```python
from build123d import *

# Parameters (mm, degrees)
SKETCH1_W              = 20
SKETCH1_H              = 50
BOSS_EXTRUDE1_DEPTH    = 15
SKETCH3_W              = 20
SKETCH3_H              = 50
BOSS_EXTRUDE2_DEPTH    = 7.5
M8X1_25_TAPPED_HOLE1_D = 6.8


with BuildPart() as part:
    # Sketch1 → Boss-Extrude1 (new body)
    with BuildSketch(Plane(origin=(0, 0, 0), x_dir=(1, 0, 0), z_dir=(0, 1, 0))):
        with Locations((10, 25)):
            Rectangle(SKETCH1_W, SKETCH1_H)
    extrude(amount=BOSS_EXTRUDE1_DEPTH)

    # Sketch3 → Boss-Extrude2 (add)
    with BuildSketch(Plane(origin=(0, 0, 0), x_dir=(-1, 0, 0), z_dir=(0, -1, 0))):
        with Locations((-30, 25)):
            Rectangle(SKETCH3_W, SKETCH3_H)
    extrude(amount=-BOSS_EXTRUDE2_DEPTH)

    # M8x1.25 Tapped Hole1 (through all)
    with Locations(Plane(origin=(0, 15, 0), x_dir=(1, 0, 0), z_dir=(0, 1, 0))):
        with Locations((10, 25)):
            Hole(M8X1_25_TAPPED_HOLE1_D / 2)


solid = part.part
```
Source: CAD feature listing. Evaluate the final solid. Frame: model axes, mm. A direction names the side the tool comes from. Give positions to 0.01 mm unless a question says otherwise; leave off trailing zeros. Loops run counter-clockwise (first coordinate to the right, second up) from the corner with the lowest first, then second, coordinate; pieces in that order, holes last. Notation, with made-up numbers: (60, -1.75) -> (109, -1.75) arc R13 ccw to (109, 2.25) -> close; hole circle Ø4 at (-12.5, 79.5). An arc over 180 degrees is marked (long way). Put each result on its own line as item: value. Start each with the question number.
1) Material intervals for probe 1 along X at (y, z) = (4, -25); probe 2 along Z at (x, y) = (10, 4.75); probe 3 along X at (y, z) = (7.75, -25), sorted ascending.
2) Cut plane B-B (x = 10). Return loops of the section in (y, z), then the cut area to 3 significant figures.
3) Draft query along X for faces 1 (the face through (40, 4, -25)), 2 (the face through (16, 6, -50)), 3 (the face through (0, 7, -25)), 4 (the face through (8.172, 7.395, -27.867)). Return one class per face: released by +X, released by -X, zero draft, split by the parting line, or undercut.
4) Cut plane A-A (z = -25). Return loops of the section in (x, y).
5) Cut plane D-D (y = 2.5). Return loops of the section in (x, z).
6) Contact query for flat-ended pins moving along their axis: P1, Ø6, axis at y = 12.5, z = -36, coming from the +X side; P2, Ø6, axis at x = 33, z = -16.5, coming from the +Y side. Output: stop coordinate, or through.
7) Cut plane C-C (y = 10.25). Return loops of the section in (x, z), then the cut area to 3 significant figures.
8) Reachability of faces 5 (the face through (20, 11, -25)), 6 (the face through (20, 0, -25)) from +Z, -Z, +X, -X, +Y, -Y: full face, straight path, thin tool, end or side. Return the list, or none.
Results are:
1. probe 1: x = 0 to 6.6, 13.4 to 40
1. probe 2: z = -50 to -28.4, -21.6 to 0
1. probe 3: x = 0 to 6.6, 13.4 to 20
2. outline: (0, -50) -> (15, -50) -> (15, -28.4) -> (0, -28.4) -> close; (0, -21.6) -> (15, -21.6) -> (15, 0) -> (0, 0) -> close
2. area: 648 mm2
3. face 1: released by +X
3. face 2: zero draft
3. face 3: released by -X
3. face 4: undercut
4. outline: (0, 0) -> (6.6, 0) -> (6.6, 15) -> (0, 15) -> close; (13.4, 0) -> (40, 0) -> (40, 7.5) -> (20, 7.5) -> (20, 15) -> (13.4, 15) -> close
5. outline: (0, -50) -> (40, -50) -> (40, 0) -> (0, 0) -> close; hole circle Ø6.8 at (10, -25)
6. P1: stops at x = 20
6. P2: stops at y = 7.5
7. outline: (0, -50) -> (20, -50) -> (20, 0) -> (0, 0) -> close; hole circle Ø6.8 at (10, -25)
7. area: 964 mm2
8. face 5: +Z, -Z, +X, +Y
8. face 6: +Z, -Z, +X, -X, -Y
